Verification items for this drawing (mm, ordinates from the low corner). Give positions to 0.01 mm unless a question says otherwise; leave off trailing zeros. Write each loop counter-clockwise with the first axis right and the second up, starting at its lowest first coordinate (ties: lowest second). Pieces come first, ordered by that corner, then holes. Notation, with made-up numbers: (38, 70) -> (75, 70) arc R31 ccw to (75, 97) -> close; hole circle Ø10 at (65.5, -2). An arc over 180 degrees is marked (long way). Use one line per item in the form item = value. Start each with the question number.
(1) Depth check by flat-ended pin: pin 1 Ø1.5 at (x, z) = (18, 1) entering from -Y; pin 2 Ø1.5 at (x, z) = (42.5, 1.5) entering from -Y. Enter the tip coordinate at first touch or a pass-through.
(2) Section check D-D, the plane x = 4.5. Record the cut outline in (y, z).
(3) Section check C-C, the plane y = 22.5. Record the cut outline in (x, z).
(4) Section check A-A, the plane z = 0.55. Record the cut outline in (x, y), plus the area to 3 significant figures.
(5) Section check B-B, the plane x = 22.5. Record the cut outline in (y, z), plus the area to 3 significant figures.
(6) Scan lines: L1, parallel to Y at x = 22.5, z = 2.65; L2, parallel to X at y = 23.5, z = 2.25; L3, parallel to Y at x = 25, z = 0.55. Record each from-to range of solid material in increasing order.
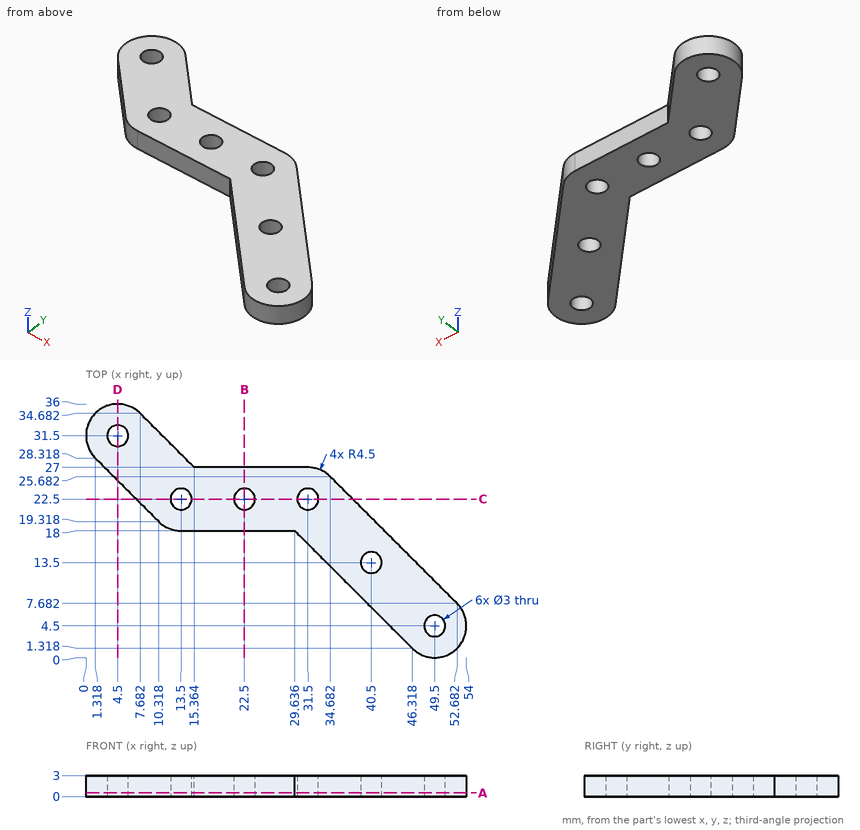
Completed:
q1.pin_1 = 18
q1.pin_2 = 4.39
q2.outline = (25.14, 0) -> (30, 0) -> (30, 3) -> (25.14, 3) -> close; (33, 0) -> (36, 0) -> (36, 3) -> (33, 3) -> close
q3.outline = (7.14, 0) -> (12, 0) -> (12, 3) -> (7.14, 3) -> close; (15, 0) -> (21, 0) -> (21, 3) -> (15, 3) -> close; (24, 0) -> (30, 0) -> (30, 3) -> (24, 3) -> close; (33, 0) -> (37.86, 0) -> (37.86, 3) -> (33, 3) -> close
q4.outline = (1.32, 28.32) -> (10.32, 19.32) arc R4.5 ccw to (13.5, 18) -> (29.64, 18) -> (46.32, 1.32) arc R4.5 ccw to (52.68, 7.68) -> (34.68, 25.68) arc R4.5 ccw to (31.5, 27) -> (15.36, 27) -> (7.68, 34.68) arc R4.5 ccw to start; hole circle Ø3 at (4.5, 31.5); hole circle Ø3 at (13.5, 22.5); hole circle Ø3 at (22.5, 22.5); hole circle Ø3 at (31.5, 22.5); hole circle Ø3 at (40.5, 13.5); hole circle Ø3 at (49.5, 4.5)
q4.area = 526 mm²
q5.outline = (18, 0) -> (21, 0) -> (21, 3) -> (18, 3) -> close; (24, 0) -> (27, 0) -> (27, 3) -> (24, 3) -> close
q5.area = 18.0 mm²
q6.L1 = 18 to 21, 24 to 27
q6.L2 = 6.14 to 12.38, 14.62 to 21.38, 23.62 to 30.38, 32.62 to 36.86
q6.L3 = 18 to 27
